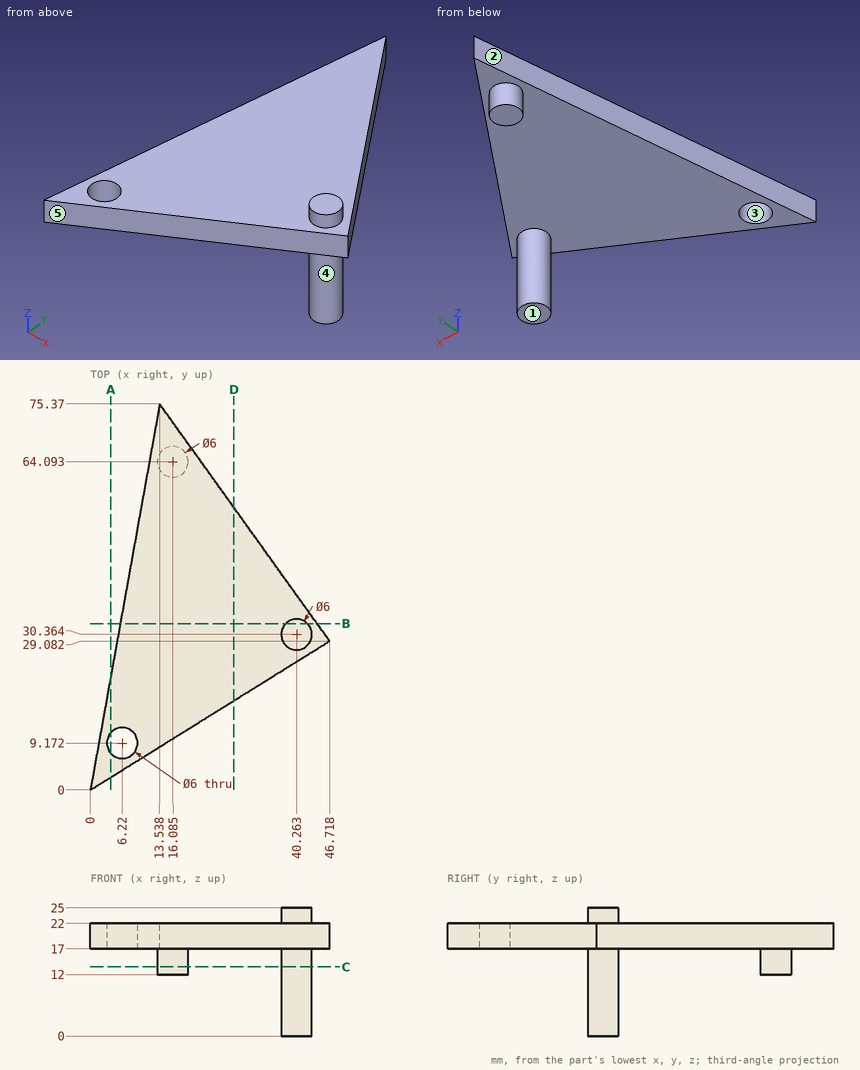
Could you check a few things on this drawing? It's one solid part, dimensions in mm from its lowest x, y, z. A direction names the side the tool comes from. Round coordinates to 2 decimals unless told otherwise and drop trailing zeros. Order: outer loops, then holes, each group sorted by start corner. A loop starts at its lowest first (then second) coordinate and runs counter-clockwise, first axis right, second up.
(1) If we mould it in two halves opening along Y, with no side actions, what happens to the marked faces 1, 2 and 3? For each: released by +Y, released by -Y, zero draft, split by the parting line, or undercut.
Response values:
face 1: zero draft
face 2: released by +Y
face 3: undercut
(2) Imagine slicing it at D-D (x = 28). Write out the boundary of the cut face in (y, z) (1 decimal), plus the area to 3 significant figures.
Response values:
outline: (17.4, 17) - (55.2, 17) - (55.2, 22) - (17.4, 22) - close
area: 189 mm2
(3) I'm going to push flat-ended pins straight in: pin 1 (12 mm diameter, centred on x = 35.5, y = 60.5, fed in from -Z); pin 2 (14 mm diameter, centred on x = 17.5, y = 50, fed in from -Z); pin 3 (12 mm diameter, centred on y = 57, z = 8.5, fed in from +X); pin 4 (1 mm diameter, centred on x = 14.5, z = 12.5, fed in from -Y). Where does each tip first touch, or does it pass through?
Response values:
pin 1: passes through
pin 2: stops at z = 17
pin 3: stops at x = 18.1
pin 4: stops at y = 61.3
(4) Imagine slicing it at B-B (y = 32.5). Write out the boundary of the cut face in (x, z).
Response values:
outline: (5.84, 17) - (38.16, 17) - (38.16, 0) - (42.37, 0) - (42.37, 17) - (44.27, 17) - (44.27, 22) - (42.37, 22) - (42.37, 25) - (38.16, 25) - (38.16, 22) - (5.84, 22) - close
(5) Which directions (+Z, -Z, +X, -X, +Y, -Y) give clear straight access to the entire face, cutting with the end or side of a thin tool? Please do the marked faces 4 and 5.
Response values:
face 4: -Z
face 5: +Z, -Z, +X, -Y
(6) Please list where these lines run through material, in increasing order: line 1 along Z through (x, y) = (28.5, 29.5); line 2 along X through (y, z) = (66, 21.5) (1 decimal); line 3 along X through (y, z) = (30.5, 2.25) (1 decimal).
Response values:
line 1: z = 17 to 22
line 2: x = 11.9 to 20.3
line 3: x = 37.3 to 43.3
(7) Imagine slicing it at C-C (z = 13.5). Write out the boundary of the cut face in (x, y) (1 decimal).
Response values:
outline: circle Ø6 at (16.1, 64.1); circle Ø6 at (40.3, 30.4)
(8) Imagine slicing it at A-A (x = 4). Write out the boundary of the cut face in (y, z).
Response values:
outline: (2.49, 17) - (7.15, 17) - (7.15, 22) - (2.49, 22) - close; (11.19, 17) - (22.27, 17) - (22.27, 22) - (11.19, 22) - close
